The listing builds one solid part. Answer for the finished solid, in the listing's coordinates (mm). A direction names the side the tool comes from. Give positions to 0.01 mm unless a question says otherwise; leave off trailing zeros. Order: outer loops, then holes, each group sorted by start corner. A loop starts at its lowest first (then second) coordinate and runs counter-clockwise, first axis right, second up. Notation, with made-up numbers: (-3, -13.75) - (19, -13.75) arc R7 ccw to (19, -1.75) - close; hole circle Ø3 at (74.25, 55.25). An arc over 180 degrees is marked (long way). Write each question's results on one line, items separated by ' | '. Start each with the question number.
1. Section D-D (x = 12.7) is taken. Give the vertices of the cut face in (y, z) (3 decimals).
2. Section B-B (y = 12.7) is taken. Give the vertices of the cut face in (x, z) (3 decimals), and give its area (3 significant figures).
3. Find the intervals of material crossed by L1, parallel to Y at x = 12.5, z = 6.25; L2, parallel to Y at x = 12.7, z = 2; L3, parallel to X at y = 13, z = 8.25, in increasing order.
4. Determine the mould class of faces 3 (the face through (25, 26, 0)), 4 (the face through (25, 50.8, 5)), 5 (the face through (25, 0, 5)), 6 (the face through (11.98, 43.61, 6.39)) for opening direction Y: released by +Y, released by -Y, zero draft, split by the parting line, or undercut.
5. Section A-A (x = 38.1) is taken. Give the vertices of the cut face in (y, z) (3 decimals), and give its area (3 significant figures).
6. Which of the six approach directions +Z, -Z, +X, -X, +Y, -Y give full straight-line access (tool end or side, diameter ignored) to faces 1 (the face through (38.653, 35.608, 4.696)), 2 (the face through (16.3, 38.2, 3.175))?
7. Section C-C (z = 5) is taken. Give the vertices of the cut face in (x, y), and give its area (3 significant figures).
8. Flat-ended cylindrical pins translate along their axes: pin 1 (4 mm diameter, centred on x = 26, z = 3, fed in from -Y); pin 2 (11 mm diameter, centred on x = 12.7, y = 38.1, fed in from +Z) (3 decimals). Find the tip coordinate at first contact, or state that the pin passes through.
from build123d import *

# Parameters (mm, degrees)
SKETCH1_W                                           = 50.8
SKETCH1_H                                           = 50.8
BOSS_EXTRUDE1_DEPTH                                 = 9.525
CBORE_FOR_1_4_SOCKET_HEAD_CAP_SCREW1_D              = 6.7564
CBORE_FOR_1_4_SOCKET_HEAD_CAP_SCREW1_CBORE_D        = 11.1125
CBORE_FOR_1_4_SOCKET_HEAD_CAP_SCREW1_CBORE_DEPTH    = 6.35
F_1_4_20_TAPPED_HOLE1_D                             = 5.1054
CSK_FOR_1_4_FLAT_HEAD_MACHINE_SCREW_100_D           = 6.7564
CSK_FOR_1_4_FLAT_HEAD_MACHINE_SCREW_100_CSINK_D     = 12.8778
CSK_FOR_1_4_FLAT_HEAD_MACHINE_SCREW_100_CSINK_ANGLE = 100


with BuildPart() as part:
    # Sketch1 → Boss-Extrude1 (new body)
    with BuildSketch(Plane.XY):
        with Locations((25.4, 25.4)):
            Rectangle(SKETCH1_W, SKETCH1_H)
    extrude(amount=BOSS_EXTRUDE1_DEPTH)

    # CBORE for 1/4 Socket Head Cap Screw1 (through all)
    with Locations(Plane.XY.offset(9.525)):
        with Locations((12.7, 38.1)):
            CounterBoreHole(CBORE_FOR_1_4_SOCKET_HEAD_CAP_SCREW1_D / 2, CBORE_FOR_1_4_SOCKET_HEAD_CAP_SCREW1_CBORE_D / 2, CBORE_FOR_1_4_SOCKET_HEAD_CAP_SCREW1_CBORE_DEPTH)

    # 1/4-20 Tapped Hole1 (through all)
    with Locations(Plane.XY.offset(9.525)):
        with Locations((38.1, 38.1), (38.1, 12.7)):
            Hole(F_1_4_20_TAPPED_HOLE1_D / 2)

    # CSK for 1/4 Flat Head Machine Screw (100)1 (through all)
    with Locations(Plane.XY.offset(9.525)):
        with Locations((12.7, 12.7)):
            CounterSinkHole(CSK_FOR_1_4_FLAT_HEAD_MACHINE_SCREW_100_D / 2, CSK_FOR_1_4_FLAT_HEAD_MACHINE_SCREW_100_CSINK_D / 2, counter_sink_angle=CSK_FOR_1_4_FLAT_HEAD_MACHINE_SCREW_100_CSINK_ANGLE)


solid = part.part
Reported:
1) outline: (0, 0) - (9.322, 0) - (9.322, 6.957) - (6.261, 9.525) - (0, 9.525) - close; (16.078, 0) - (34.722, 0) - (34.722, 3.175) - (32.544, 3.175) - (32.544, 9.525) - (19.139, 9.525) - (16.078, 6.957) - close; (41.478, 0) - (50.8, 0) - (50.8, 9.525) - (43.656, 9.525) - (43.656, 3.175) - (41.478, 3.175) - close
2) outline: (0, 0) - (9.322, 0) - (9.322, 6.957) - (6.261, 9.525) - (0, 9.525) - close; (16.078, 0) - (35.547, 0) - (35.547, 9.525) - (19.139, 9.525) - (16.078, 6.957) - close; (40.653, 0) - (50.8, 0) - (50.8, 9.525) - (40.653, 9.525) - close | area: 363 mm²
3) L1: 0 to 9.33, 16.07 to 32.55, 43.65 to 50.8 | L2: 0 to 9.32, 16.08 to 34.72, 41.48 to 50.8 | L3: 0 to 7.79, 17.61 to 35.56, 40.64 to 50.8
4) face 3: zero draft | face 4: released by +Y | face 5: released by -Y | face 6: undercut
5) outline: (0, 0) - (10.147, 0) - (10.147, 9.525) - (0, 9.525) - close; (15.253, 0) - (35.547, 0) - (35.547, 9.525) - (15.253, 9.525) - close; (40.653, 0) - (50.8, 0) - (50.8, 9.525) - (40.653, 9.525) - close | area: 387 mm²
6) face 1: +Z, -Z | face 2: +Z
7) outline: (0, 0) - (50.8, 0) - (50.8, 50.8) - (0, 50.8) - close; hole circle Ø11.11 at (12.7, 38.1); hole circle Ø6.76 at (12.7, 12.7); hole circle Ø5.11 at (38.1, 12.7); hole circle Ø5.11 at (38.1, 38.1) | area: 2,410 mm²
8) pin 1: y = 0 | pin 2: z = 3.175
